Input: part model. Units: mm. Frame: model coordinates. A direction names the side the tool comes from. Round coordinates to 2 decimals unless told otherwise and drop trailing zeros. Order: outer loops, then holes, each group sorted by start corner. A loop starts at its lowest first (then second) coordinate and runs counter-clockwise, first axis right, second up. Notation, with made-up numbers: (45, -37.75) -> (83, -37.75) arc R21 ccw to (83, -19.75) -> close; hole circle Ø11 at (79.5, -9). An arc over 180 degrees is marked (long way). Answer as CSV lines item,"result". Start each with the question number.
1) Section query C-C, the plane y = -38.5. Output: boundary loops of the cut face in (x, z), and give its area (3 significant figures).
2) Section query A-A, the plane y = -3. Output: boundary loops of the cut face in (x, z), and give its area (3 significant figures).
3) First-contact query: P1, Ø9, axis at y = 0, z = 0, coming from the +X side. Flat tip, straight axial feed; report the tip coordinate or a pass-through.
4) Section query B-B, the plane x = 1.2. Output: boundary loops of the cut face in (y, z).
5) Line query: L1, parallel to Z at x = 1.1, y = -47; L2, parallel to Y at x = 0.2, z = 8.5; L3, parallel to Z at x = 1.05, y = -42. Output: solid intervals per line, ascending.
6) Access query for faces 1 (the face through (0.783, -76.852, 5.477)), 2 (the face through (0, -9, 0)), 3 (the face through (0.783, 50.037, 5.527)). Directions: +Z, -Z, +X, -X, +Y, -Y. A direction counts if a zero-diameter tool reaches every point of the face in a straight line with its end or side. Return the directions, or none.
7) Mould query, pull axis Z, two halves, no side actions, for faces 4 (the face through (0.783, -83.144, 0.341)), 5 (the face through (0.783, -67.414, 0.602)), 6 (the face through (1.588, -9, 0)). Classes: +Z half, -Z half, draft (parallel to the pull), parting line (faces both ways), or undercut.
```python
from build123d import *

# Parameters (mm, degrees)
SKETCH1_R           = 7.62
BOSS_EXTRUDE1_DEPTH = 1.5875


with BuildPart() as part:
    # Sketch1 → Boss-Extrude1 (new body)
    with BuildSketch(Plane(origin=(0, 0, 0), x_dir=(0, 0, -1), z_dir=(1, 0, 0))):
        with BuildLine():
            Line((-12.642487664, 65.178590664), (-12.468624959, 55.244460434))
            Line((-12.468624959, 55.244460434), (-3.075732618, 60.888873679))
            ThreePointArc((-3.075732618, 60.888873679), (2.439979404, 59.513924484), (1.065030209, 53.998212461))
            Line((1.065030209, 53.998212461), (-12.306187241, 45.963128683))
            Line((-12.306187241, 45.963128683), (-10.108033982, -79.634484144))
            Line((-10.108033982, -79.634484144), (-0.715141642, -73.990070899))
            ThreePointArc((-0.715141642, -73.990070899), (4.800570381, -75.365020094), (3.425621185, -80.880732117))
            Line((3.425621185, -80.880732117), (-4.214042055, -85.47158814))
            Line((-4.214042055, -85.47158814), (12.992376231, -85.170449101))
            Line((12.992376231, -85.170449101), (10.353990645, 65.581064744))
            Line((10.353990645, 65.581064744), (-12.642487664, 65.178590664))
        make_face()
        with Locations((-0.699777134, 39.983716876)):
            Circle(SKETCH1_R, mode=Mode.SUBTRACT)
        with Locations((-0.349888567, 19.991858438)):
            Circle(SKETCH1_R, mode=Mode.SUBTRACT)
        Circle(SKETCH1_R, mode=Mode.SUBTRACT)
        with Locations((0.349888567, -19.991858438)):
            Circle(SKETCH1_R, mode=Mode.SUBTRACT)
        with Locations((0.699777134, -39.983716876)):
            Circle(SKETCH1_R, mode=Mode.SUBTRACT)
        with Locations((1.049665701, -59.975575313)):
            Circle(SKETCH1_R, mode=Mode.SUBTRACT)
    extrude(amount=BOSS_EXTRUDE1_DEPTH)


solid = part.part
```
Findings:
1,outline,"(0, -12.18) -> (1.59, -12.18) -> (1.59, -8.17) -> (0, -8.17) -> close; (0, 6.77) -> (1.59, 6.77) -> (1.59, 10.83) -> (0, 10.83) -> close"
1,area,"12.8 mm^2"
2,outline,"(0, -11.55) -> (1.59, -11.55) -> (1.59, -7) -> (0, -7) -> close; (0, 7) -> (1.59, 7) -> (1.59, 11.45) -> (0, 11.45) -> close"
2,area,"14.3 mm^2"
3,P1,"passes through"
4,outline,"(-85.47, 4.21) -> (-85.17, -12.99) -> (65.58, -10.35) -> (65.18, 12.64) -> (55.24, 12.47) -> (60.89, 3.08) arc R4.02 cw to (54, -1.07) -> (45.96, 12.31) -> (-79.63, 10.11) -> (-73.99, 0.72) arc R4.02 cw to (-80.88, -3.43) -> close; hole circle Ø15.24 at (-59.98, -1.05); hole circle Ø15.24 at (-39.98, -0.7); hole circle Ø15.24 at (-19.99, -0.35); hole circle Ø15.24 at (0, 0); hole circle Ø15.24 at (19.99, 0.35); hole circle Ø15.24 at (39.98, 0.7)"
5,L1,"z = -12.32 to -3.67, 2.27 to 10.68"
5,L2,"y = -78.67 to 48.25, 57.63 to 65.25"
5,L3,"z = -12.24 to -8.05, 6.65 to 10.77"
6,face 1,"+X, -X"
6,face 2,"+Z, -Z, -X, +Y, -Y"
6,face 3,"+Z, +X, -X"
7,face 4,"+Z half"
7,face 5,"undercut"
7,face 6,"draft"
